```python
from build123d import *

# Parameters (mm, degrees)
SKETCH015_R     = 2.15
SKETCH015_R_2   = 1.6
PAD005_DEPTH    = 15
FILLET003_R     = 3
FILLET004_R     = 2
CHAMFER007_SIZE = 1
SKETCH016_R     = 2.1
SKETCH016_W     = 16
SKETCH016_H     = 8.2
POCKET008_DEPTH = 18.001
POCKET009_DEPTH = 9
FILLET005_R     = 2
POCKET010_DEPTH = 18.001
FILLET006_R     = 0.3


with BuildPart() as part:
    # Sketch015 (on Face1 of Binder001) → Pad005 (new body)
    with BuildSketch(Plane(origin=(1.2e-05, -73, 0), x_dir=(1, 0, 0), z_dir=(0, -1, 0))):
        Polygon((-29.75, 93), (-29.75, 111), (29.75, 111), (29.75, 93), (17.75, 93), (17.75, 99), (-17.75, 99), (-17.75, 93), align=None)
        with Locations((-25.75, 106.751)):
            Circle(SKETCH015_R, mode=Mode.SUBTRACT)
        with Locations((-25.75, 97)):
            Circle(SKETCH015_R_2, mode=Mode.SUBTRACT)
        with Locations((25.75, 97)):
            Circle(SKETCH015_R_2, mode=Mode.SUBTRACT)
        with Locations((25.75, 106.751)):
            Circle(SKETCH015_R, mode=Mode.SUBTRACT)
    extrude(amount=PAD005_DEPTH)

    # Fillet003
    fillet003_edges = [part.edges().sort_by_distance(p)[0] for p in [
        (-29.749986, -80.500005, 111),
        (29.750014, -80.499995, 111),
        (-29.749986, -80.500005, 93),
        (-17.749986, -80.500003, 93),
        (17.750014, -80.499997, 93),
        (29.750014, -80.499995, 93),
    ]]
    fillet(fillet003_edges, radius=FILLET003_R)

    # Fillet004
    fillet004_edges = [part.edges().sort_by_distance(p)[0] for p in [
        (-17.749986, -80.500003, 99),
        (17.750014, -80.499997, 99),
    ]]
    fillet(fillet004_edges, radius=FILLET004_R)

    # Chamfer007
    chamfer007_edges = [part.edges().sort_by_distance(p)[0] for p in [
        (23.600012, -72.999996, 106.751),
        (24.150012, -72.999996, 97),
        (-27.349988, -73.000005, 97),
        (-27.899988, -73.000005, 106.751),
        (24.150015, -87.999996, 97),
        (23.600015, -87.999996, 106.751),
        (-27.899985, -88.000005, 106.751),
        (-27.349985, -88.000005, 97),
    ]]
    chamfer(chamfer007_edges, length=CHAMFER007_SIZE)

    # Sketch016 (on Face15 of Chamfer007) → Pocket008 (cut, through all)
    with BuildSketch(Plane.XY.offset(111)):
        with Locations((-10.5, -80.5)):
            Circle(SKETCH016_R)
        with Locations((10.5, -80.5)):
            Circle(SKETCH016_R)
        with Locations((0, -80.5)):
            Rectangle(SKETCH016_W, SKETCH016_H)
    extrude(amount=-POCKET008_DEPTH, mode=Mode.SUBTRACT)

    # Sketch017 (on Face6 of Pocket008) → Pocket009 (cut)
    with BuildSketch(Plane(origin=(0, 0, 99), x_dir=(1, 0, 0), z_dir=(0, 0, -1))):
        with BuildLine():
            ThreePointArc((-10.5, 85.1), (-15.1, 80.5), (-10.5, 75.9))
            Line((-10.5, 75.9), (10.5, 75.9))
            ThreePointArc((10.5, 75.9), (15.1, 80.5), (10.5, 85.1))
            Line((10.5, 85.1), (-10.5, 85.1))
        make_face()
    extrude(amount=-POCKET009_DEPTH, mode=Mode.SUBTRACT)

    # Fillet005
    fillet005_edges = [part.edges().sort_by_distance(p)[0] for p in [
        (-8, -76.4, 109.5),
        (-8, -84.6, 109.5),
    ]]
    fillet(fillet005_edges, radius=FILLET005_R)

    # Sketch018 (on Face1 of Fillet005) → Pocket010 (cut, through all)
    with BuildSketch(Plane.XY.offset(111)):
        with BuildLine():
            ThreePointArc((-10.5, -79.5), (-11.5, -80.5), (-10.5, -81.5))
            Line((-10.5, -81.5), (10.5, -81.5))
            ThreePointArc((10.5, -81.5), (11.5, -80.5), (10.5, -79.5))
            Line((10.5, -79.5), (-10.5, -79.5))
        make_face()
    extrude(amount=-POCKET010_DEPTH, mode=Mode.SUBTRACT)

    # Fillet006
    fillet006_edges = [part.edges().sort_by_distance(p)[0] for p in [
        (-8, -79.5, 109.5),
        (-8.653381, -79.5, 109.5),
        (-8, -81.5, 109.5),
        (-8.653381, -81.5, 109.5),
        (8.653381, -79.5, 109.5),
        (8, -79.5, 109.5),
        (8.653381, -81.5, 109.5),
        (8, -81.5, 109.5),
    ]]
    fillet(fillet006_edges, radius=FILLET006_R)


solid = part.part
```
The model under review builds one solid part; all positions refer to its coordinate system, in mm. A direction names the side the tool comes from. Round coordinates to 2 decimals unless told otherwise and drop trailing zeros. Order: outer loops, then holes, each group sorted by start corner. A loop starts at its lowest first (then second) coordinate and runs counter-clockwise, first axis right, second up. Notation, with made-up numbers: (74.25, 23) -> (104.25, 23) arc R22 ccw to (104.25, 39) -> close; hole circle Ø3 at (9.5, 3). An arc over 180 degrees is marked (long way). Use a Markdown table: item, result.
Q1. Tool access review of faces 5 (the cylindrical face through (-26.03, -80.409, 108.883)), 6 (the flat face through (8, -83, 110)), 7 (the cylindrical face through (-17.18, -80.6, 98.4)), 8 (the flat face through (0, -85.1, 103)): name each direction out of +Z, -Z, +X, -X, +Y, -Y from which nothing blocks a thin tool from reaching the whole face with its end or side.
Values:
| item | result |
|---|---|
| face 5 | +Y, -Y |
| face 6 | +Z, -Z |
| face 7 | -Z, +Y, -Y |
| face 8 | -Z |
Q2. We need section A-A on x = 5.5. Write out the cut boundary in (y, z), then the cut area to 3 significant figures.
Values:
| item | result |
|---|---|
| outline | (-88, 99) -> (-85.1, 99) -> (-85.1, 108) -> (-84.6, 108) -> (-84.6, 111) -> (-88, 111) -> close; (-76.4, 108) -> (-75.9, 108) -> (-75.9, 99) -> (-73, 99) -> (-73, 111) -> (-76.4, 111) -> close |
| area | 72.6 mm^2 |
Q3. We need section C-C on y = -83.75. Write out the cut boundary in (x, z), then the cut area to 3 significant figures.
Values:
| item | result |
|---|---|
| outline | (-29.75, 96) arc R3 ccw to (-26.75, 93) -> (-20.75, 93) arc R3 ccw to (-17.75, 96) -> (-17.75, 97) arc R2 cw to (-15.75, 99) -> (-13.76, 99) -> (-13.76, 108) -> (-7.64, 108) -> (-7.64, 111) -> (-26.75, 111) arc R3 ccw to (-29.75, 108) -> close; (8, 108) -> (13.76, 108) -> (13.76, 99) -> (15.75, 99) arc R2 cw to (17.75, 97) -> (17.75, 96) arc R3 ccw to (20.75, 93) -> (26.75, 93) arc R3 ccw to (29.75, 96) -> (29.75, 108) arc R3 ccw to (26.75, 111) -> (8, 111) -> close; hole circle Ø4.3 at (-25.75, 106.75); hole circle Ø3.2 at (-25.75, 97); hole circle Ø4.3 at (25.75, 106.75); hole circle Ø3.2 at (25.75, 97) |
| area | 508 mm^2 |
Q4. Mouldability with a two-part tool opening along Z and no side actions: class faces 1 (the cylindrical face through (24.15, -80.41, 97.07)), 2 (the flat face through (8, -78, 110)), 3 (the cylindrical face through (28.89, -80.6, 93.9)), 4 (the cylindrical face through (25.47, -80.409, 108.883)) as +Z half, -Z half, draft (parallel to the pull), parting line (faces both ways), or undercut.
Values:
| item | result |
|---|---|
| face 1 | undercut |
| face 2 | draft |
| face 3 | -Z half |
| face 4 | undercut |
Q5. We need section B-B on y = -80.5. Write out the cut boundary in (x, z), then the cut area to 3 significant figures.
Values:
| item | result |
|---|---|
| outline | (-29.75, 96) arc R3 ccw to (-26.75, 93) -> (-20.75, 93) arc R3 ccw to (-17.75, 96) -> (-17.75, 97) arc R2 cw to (-15.75, 99) -> (-15.1, 99) -> (-15.1, 108) -> (-12.6, 108) -> (-12.6, 111) -> (-26.75, 111) arc R3 ccw to (-29.75, 108) -> close; (12.6, 108) -> (15.1, 108) -> (15.1, 99) -> (15.75, 99) arc R2 cw to (17.75, 97) -> (17.75, 96) arc R3 ccw to (20.75, 93) -> (26.75, 93) arc R3 ccw to (29.75, 96) -> (29.75, 108) arc R3 ccw to (26.75, 111) -> (12.6, 111) -> close; hole circle Ø4.3 at (-25.75, 106.75); hole circle Ø3.2 at (-25.75, 97); hole circle Ø4.3 at (25.75, 106.75); hole circle Ø3.2 at (25.75, 97) |
| area | 456 mm^2 |
Q6. We need section D-D on y = -86. Write out the cut boundary in (x, z).
Values:
| item | result |
|---|---|
| outline | (-29.75, 96) arc R3 ccw to (-26.75, 93) -> (-20.75, 93) arc R3 ccw to (-17.75, 96) -> (-17.75, 97) arc R2 cw to (-15.75, 99) -> (15.75, 99) arc R2 cw to (17.75, 97) -> (17.75, 96) arc R3 ccw to (20.75, 93) -> (26.75, 93) arc R3 ccw to (29.75, 96) -> (29.75, 108) arc R3 ccw to (26.75, 111) -> (-26.75, 111) arc R3 ccw to (-29.75, 108) -> close; hole circle Ø4.3 at (-25.75, 106.75); hole circle Ø3.2 at (-25.75, 97); hole circle Ø4.3 at (25.75, 106.75); hole circle Ø3.2 at (25.75, 97) |
Q7. For line 1 (X direction, y = -82.25, z = 97.25); line 2 (Y direction, x = -4, z = 104.25); line 3 (X direction, y = -81.5, z = 96.75), list the stretches that pass through material, from the lowest coordinate up.
Values:
| item | result |
|---|---|
| line 1 | x = -29.75 to -27.33, -24.17 to -17.73, 17.73 to 24.17, 27.33 to 29.75 |
| line 2 | y = -88 to -85.1, -75.9 to -73 |
| line 3 | x = -29.75 to -27.33, -24.17 to -17.75, 17.75 to 24.17, 27.33 to 29.75 |
Q8. Clearance check with flat-ended pins moving along their axes: P1, Ø6.5, axis at x = 10.5, y = -80.5, coming from the +Z side; P2, Ø1.4, axis at y = -77, z = 110, coming from the -X side; P3, Ø8, axis at x = 8, y = -84, coming from the -Z side; P4, Ø2, axis at y = -83.5, z = 109.5, coming from the -X side. State where each tip first meets the part, or that it passes through.
Values:
| item | result |
|---|---|
| P1 | stops at z = 111 |
| P2 | stops at x = -29.45 |
| P3 | stops at z = 99 |
| P4 | stops at x = -29.71 |
